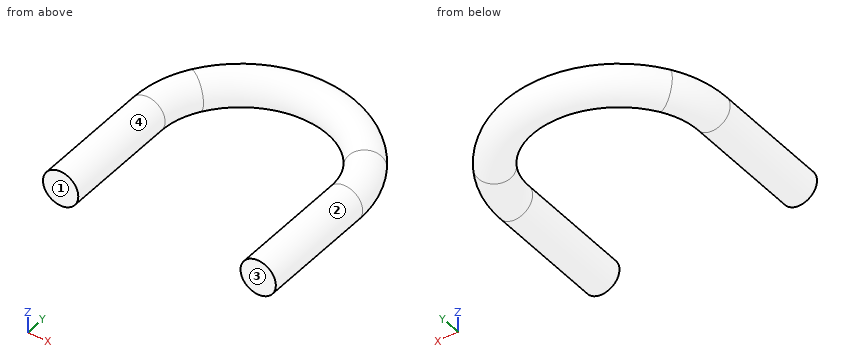
from build123d import *

# Parameters (mm, degrees)
SWEEP1_OUTLINE_R   = 5
SWEEP1_DEPTH       = 33.988332717
SWEEP1_2_OUTLINE_R = 5
SWEEP1_2_ANGLE     = 32.92809
SWEEP1_3_OUTLINE_R = 5
SWEEP1_3_ANGLE     = 114.14382
SWEEP1_4_OUTLINE_R = 5
SWEEP1_4_ANGLE     = 32.92809
SCALE7_SCALE       = 2.5


with BuildPart() as part:
    # Sweep1: read off the stored shape, not the designer's step
    # Sweep1 outline → Sweep1 (new body)
    with BuildSketch(Plane(origin=(0, 0, 0), x_dir=(1, 0, 0), z_dir=(0, 1, 0))):
        with Locations((55.902877487, 0)):
            Circle(SWEEP1_OUTLINE_R)
        Circle(SWEEP1_OUTLINE_R)
    extrude(amount=SWEEP1_DEPTH)



with BuildPart() as body_2:
    # Sweep1 2 outline → Sweep1 2 (revolve)
    with BuildSketch(Plane(origin=(31.307900209, 33.988332717, 0), x_dir=(1, 0, 0), z_dir=(0, -1, 0))):
        with Locations((24.594977278, 0)):
            Circle(SWEEP1_2_OUTLINE_R)
    revolve(axis=Axis((31.307900209, 33.988332717, 0), (0, 0, 1)), revolution_arc=SWEEP1_2_ANGLE)

    # Sweep1 3 outline → Sweep1 3 (revolve)
    with BuildSketch(Plane(origin=(27.951438743, 31.814605451, 0), x_dir=(0.8393534671240316, 0.5435860164011462, 0), z_dir=(0.5435860164011462, -0.8393534671240316, 0))):
        with Locations((28.593842592, 0)):
            Circle(SWEEP1_3_OUTLINE_R)
    revolve(axis=Axis((27.951438743, 31.814605451, 0), (0, 0, 1)), revolution_arc=SWEEP1_3_ANGLE)


with BuildPart() as part_1:
    add(part.part)

    add(body_2.part)  # Sweep1 4 merges body 2
    # Sweep1 4 outline → Sweep1 4 (revolve)
    with BuildSketch(Plane(origin=(24.594977278, 33.988332717, 0), x_dir=(-0.8393534671240301, 0.5435860164011485, 0), z_dir=(0.5435860164011485, 0.8393534671240301, 0))):
        with Locations((24.594977278, 0)):
            Circle(SWEEP1_4_OUTLINE_R)
    revolve(axis=Axis((24.594977278, 33.988332717, 0), (0, 0, 1)), revolution_arc=SWEEP1_4_ANGLE)


with BuildPart() as part_2:
    # Scale7: scaled about (27.951438772, 35.9486859, 0)
    add(part_1.part.scale(SCALE7_SCALE).moved(Location((-41.927158158, -53.92302885, 0))))


solid = part_2.part
Check sheet for the modelled part. Datum: model origin and axes. Units: mm. Face numbers are marked on the shaded views. A direction names the side the tool comes from. Coordinates: 2 decimals unless noted, no trailing zeros. Write each loop counter-clockwise with the first axis right and the second up, starting at its lowest first coordinate (ties: lowest second). Pieces come first, ordered by that corner, then holes. Notation, with made-up numbers: M 24,54.25 L 78,54.25 A20 ccw 78,73.25 Z; hole C 57.5,-24 d9. An arc over 180 degrees is marked long. Answer as CSV lines item,"result".
Q1. Set-up check for the marked faces 3 and 4: record each of +Z, -Z, +X, -X, +Y, -Y from which the full face is reachable in a straight line by a thin tool's end or side.
Check result:
face 3,"+Z, -Z, +X, -X, -Y"
face 4,"-Y"
Q2. Cross-section at B-B (z = 0). Record the boundary of the cut face in (x, y).
Check result:
outline,"M -54.43,-53.92 L -29.43,-53.92 L -29.43,31.05 A48.99 cw -21.56,57.68 A58.98 cw 77.46,57.68 A48.99 cw 85.33,31.05 L 85.33,-53.92 L 110.33,-53.92 L 110.33,31.05 A73.99 ccw 98.44,71.27 A83.98 ccw -42.54,71.27 A73.99 ccw -54.43,31.05 Z"
Q3. Cross-section at A-A (y = -39.5). Record the boundary of the cut face in (x, z).
Check result:
outline,"C -41.93,0 d25; C 97.83,0 d25"
Q4. Go/stop test with flat-tipped pins: pin 1 (2 mm diameter, centred on x = 69.5, z = 7, fed in from +Y); pin 2 (4 mm diameter, centred on x = -24, z = 0.5, fed in from +Y); pin 3 (2 mm diameter, centred on y = 75, z = -6.5, fed in from -X); pin 4 (6 mm diameter, centred on y = 18.5, z = -1.5, fed in from +X). Record where each tip stops, or that it passes through.
Check result:
pin 1,"y = 97.05"
pin 2,"y = 93.12"
pin 3,"x = -38.73"
pin 4,"x = 110.33"
Q5. Material ranges on probe 1 along Z at (x, y) = (-42.5, 2.5); probe 2 along X at (y, z) = (58, 3); probe 3 along X at (y, z) = (58, 1.5), recorded low to high. Write a range as from..to.
Check result:
probe 1,"-12.49..12.49"
probe 2,"-48.95..-21.78, 77.69..104.85"
probe 3,"-49.25..-21.45, 77.36..105.15"
Q6. Mould release check, pull along X, two halves, no side actions. Record for the marked faces 1 and 2: released by +X, released by -X, zero draft, split by the parting line, or undercut.
Check result:
face 1,"zero draft"
face 2,"undercut"
